Here's how the part is built. I have some questions about the finished solid (model axes, mm). A direction names the side the tool comes from. Coordinates: 2 decimals unless noted, no trailing zeros. Loops run counter-clockwise (first coordinate to the right, second up) from the corner with the lowest first, then second, coordinate; pieces in that order, holes last. Notation, with made-up numbers: M 56.25,-26 L 81.25,-26 A21 ccw 81.25,-9 Z; hole C -19.5,18.5 d6. An arc over 180 degrees is marked long. Use one line per item in the form item = value. Start each with the question number.
(1) Imagine slicing it at D-D, the plane x = 502.5. Please give me the cut outline in (y, z) (3 decimals), and give its area (3 significant figures).
(2) Imagine slicing it at A-A, the plane z = -13. Please give me the cut outline in (x, y).
(3) Will these pins go through, and if not, where does the flat tip stop? P1, Ø8, axis at x = 426, z = 5, coming from the +Y side; P2, Ø2, axis at y = 559.5, z = -147, coming from the -X side; P3, Ø3, axis at x = 327, y = 431, coming from the -Z side.
(4) Imagine slicing it at C-C, the plane z = -167. Please give me the cut outline in (x, y).
(5) Imagine slicing it at B-B, the plane y = 667. Please give me the cut outline in (x, z), and give its area (3 significant figures).
(6) On a 3-axis mill with a long thin cutter (end or side, diameter ignored), from which of +Z, -Z, +X, -X, +Y, -Y can I reach the whole of each face in a straight line? I mean faces 1 (the flat face through (720.011, 589, -91)), 2 (the cylindrical face through (398.471, 430.215, 8.073)). Say none if no direction works.
(7) Please list where these lines run through material, in increasing order: L1, parallel to X at y = 453.5, z = -70; L2, parallel to Z at x = 295.5, y = 593; L3, parallel to Z at x = 147.5, y = 420.
Autodesk Inventor part; units mm, degrees
ref_plane "YZ Plane" through (0, 0, 0) normal (1, 0, 0) x (0, 1, 0)
ref_plane "XZ Plane" through (0, 0, 0) normal (0, 1, 0) x (-1, 0, 0)
ref_plane "XY Plane" through (0, 0, 0) normal (0, 0, 1) x (1, 0, 0)
ref_plane "작업 평면1" through (0, 0.7157, 0) normal (0, 0, 1) x (1, 0, 0)
sketch "스케치1" plane through (0, 0.7157, 0) normal (0, 0, 1) x (1, 0, 0)
  line L0 (70.0112, 388.9292) -> (730.0112, 388.9292)
  line L1 (730.0112, 388.9292) -> (730.0112, 718.9292)
  line L2 (730.0112, 718.9292) -> (70.0112, 718.9292)
  line L3 (70.0112, 718.9292) -> (70.0112, 388.9292)
  point P0 (0, -0.7157)
  dimension "d0" = 660
  dimension "d1" = 330
extrude "돌출1" add sketch "스케치1" along normal blind 10
sketch "스케치2" plane through (0, 0.7157, 0) normal (0, 0, -1) x (-1, 0, 0)
  line L0 (-70.0112, 388.9292) -> (-730.0112, 388.9292)
  line L1 (-730.0112, 388.9292) -> (-720.0112, 388.9292)
  line L2 (-720.0112, 388.9292) -> (-720.0112, 478.9292)
  line L3 (-720.0112, 478.9292) -> (-730.0112, 478.9292)
  line L4 (-730.0112, 478.9292) -> (-730.0112, 388.9292)
  line L5 (-70.0112, 388.9292) -> (-80.0112, 388.9292)
  line L6 (-80.0112, 388.9292) -> (-80.0112, 478.9292)
  line L7 (-80.0112, 478.9292) -> (-70.0112, 478.9292)
  line L8 (-70.0112, 478.9292) -> (-70.0112, 388.9292)
  point P0 (0, -0.7157)
  dimension "d4" = 10
  dimension "d5" = 90
  dimension "d6" = 10
  dimension "d7" = 90
extrude "돌출2" add sketch "스케치2" along normal blind 90
fillet "모깎기1" radius 45 4 edges at (725.0112, 479.645, -90) (725.0112, 389.645, -90) (75.0112, 479.645, -90) (75.0112, 389.645, -90)
fillet "모깎기2" radius 55 1 edges at (400.0112, 389.645, 10)
sketch "스케치3" plane through (730.0112, 719.645, 10) normal (1, 0, 0) x (0, 0, -1)
  line L0 (10, -240) -> (10, 0)
  arc A0 (247.7061, -77.4327) -> (10, 0) centre (14.4307, -389.9748) ccw
  line L1 (10, 0) -> (10, -240)
  line L2 (247.7061, -77.4327) -> (91.8862, -259.2239)
  arc A1 (55, -330) -> (55, -240) centre (55, -285) ccw
  line L3 (10, -240) -> (55, -240)
  line L4 (10, -240) -> (55, -240)
  arc A2 (91.8862, -259.2239) -> (55, -240) centre (55, -285) ccw
  point P0 (10, -719.645)
  dimension "d12" = 250
  dimension "d13" = 390
extrude "돌출3" add sketch "스케치3" against normal blind 10
sketch "스케치4" plane through (70.0112, 719.645, 0) normal (-1, 0, 0) x (0, 0, 1)
  line L0 (-237.7061, -77.4327) -> (-81.8862, -259.2239)
  line L1 (-237.7061, -77.4327) -> (-81.8862, -259.2239)
  line L2 (0, 0) -> (10, 0)
  arc A0 (0, 0) -> (-237.7061, -77.4327) centre (-4.4307, -389.9748) ccw
  line L3 (0, 0) -> (0, -240)
  line L4 (0, 0) -> (0, -240)
  arc A1 (-45, -240) -> (-45, -330) centre (-45, -285) ccw
  line L5 (0, -240) -> (-45, -240)
  arc A2 (-45, -240) -> (-81.8862, -259.2239) centre (-45, -285) ccw
  point P0 (0, -719.645)
extrude "돌출4" add sketch "스케치4" against normal blind 10
sketch "스케치5" plane through (730.0112, 444.645, 10) normal (1, 0, 0) x (0, 0, -1)
  arc A0 (55, -55) -> (91.8862, 15.7761) centre (55, -10) ccw
  circle A1 centre (55, -10) radius 5
  point P0 (10, -444.645)
  dimension "d18" = 10
extrude "돌출5" add sketch "스케치5" along normal blind 10
sketch "스케치6" plane through (70.0112, 444.645, 10) normal (-1, 0, 0) x (0, 0, 1)
  arc A0 (-91.8862, 15.7761) -> (-55, -55) centre (-55, -10) ccw
  circle A1 centre (-55, -10) radius 5
  point P0 (-10, -444.645)
extrude "돌출6" add sketch "스케치6" along normal blind 10
properties part number "앞문"
Answer:
q1.outline = M 413.022,0 L 719.645,0 L 719.645,10 L 444.645,10 A55 ccw Z
q1.area = 2,960 mm²
q2.outline = M 70.01,399.91 L 80.01,399.91 L 80.01,719.58 L 70.01,719.58 Z; M 720.01,399.91 L 730.01,399.91 L 730.01,719.58 L 720.01,719.58 Z
q3.P1 = 719.64
q3.P2 = 70.01
q3.P3 = 0
q4.outline = M 70.01,559.72 L 80.01,559.72 L 80.01,684.17 L 70.01,684.17 Z; M 720.01,559.72 L 730.01,559.72 L 730.01,684.17 L 720.01,684.17 Z
q5.outline = M 70.01,-200.16 L 80.01,-200.16 L 80.01,0 L 720.01,0 L 720.01,-200.16 L 730.01,-200.16 L 730.01,10 L 70.01,10 Z
q5.area = 10,600 mm²
q6.face_1 = -Z, +Y, -Y
q6.face_2 = +Z, +X, -X, -Y
q7.L1 = 70.01 to 80.01, 720.01 to 730.01
q7.L2 = 0 to 10
q7.L3 = 0 to 4.17
